from build123d import *

# Parameters (mm, degrees)
BOSS_EXTRUDE1_DEPTH     = 68.58
CUT_EXTRUDE1_START      = -6.35
SKETCH2_R               = 21.082
CUT_EXTRUDE1_DEPTH      = 6.35
CUT_EXTRUDE2_START      = -6.35
CUT_EXTRUDE2_DEPTH      = 6.35
CUT_EXTRUDE3_DEPTH      = 93.044076876
CUT_EXTRUDE3_DEPTH_BACK = 93.044076876
FILLET1_R               = 1.27
CUT_EXTRUDE6_START      = 31.496
SKETCH8_R               = 21.082
CUT_EXTRUDE6_DEPTH      = 31.496
SKETCH9_R               = 12.7
CUT_EXTRUDE7_DEPTH      = 117.864914259
FILLET7_R               = 1.27
FILLET8_START           = 30.734
FILLET8_DEPTH           = 31.496
FILLET9_R               = 0.762
FILLET10_R              = 0.762
SKETCH10_R              = 11.6205
CUT_EXTRUDE8_DEPTH      = 29.718
SKETCH11_R              = 9.2075
CUT_EXTRUDE9_DEPTH      = 42.418


with BuildPart() as part:
    # Sketch1 → Boss-Extrude1 (new body)
    with BuildSketch(Plane(origin=(0, 0, 0), x_dir=(0, 0, -1), z_dir=(1, 0, 0))):
        with BuildLine():
            Line((-21.082, 0), (-21.082, -36.576))
            ThreePointArc((-21.082, -36.576), (0, -57.658), (21.082, -36.576))
            Line((21.082, -36.576), (21.082, 0))
            ThreePointArc((21.082, 0), (0, 21.082), (-21.082, 0))
        make_face()
    extrude(amount=BOSS_EXTRUDE1_DEPTH)

    # Sketch2 → Cut-Extrude1 (cut)
    with BuildSketch(Plane(origin=(68.58, 0, 0), x_dir=(0, 0, -1), z_dir=(1, 0, 0)).offset(CUT_EXTRUDE1_START)):
        Circle(SKETCH2_R)
    extrude(amount=CUT_EXTRUDE1_DEPTH, mode=Mode.SUBTRACT)

    # Sketch3 → Cut-Extrude2 (cut)
    with BuildSketch(Plane(origin=(68.58, 0, 0), x_dir=(0, 0, -1), z_dir=(1, 0, 0)).offset(CUT_EXTRUDE2_START)):
        with BuildLine():
            Line((-21.082, 0), (-21.082, -12.967513736))
            Line((-21.082, -12.967513736), (-17.956950774, -11.045299584))
            ThreePointArc((-17.956950774, -11.045299584), (-20.285698906, -5.739437593), (-21.082, 0))
        make_face()
    cut_extrude2 = extrude(amount=CUT_EXTRUDE2_DEPTH, mode=Mode.SUBTRACT)

    # Mirror2: Cut-Extrude2 across plane
    add(cut_extrude2.mirror(Plane.XY), mode=Mode.SUBTRACT)

    # Sketch4 → Cut-Extrude3 (cut, two sides: drawn at the far end of the back side and taken through both)
    with BuildSketch(Plane.XY.offset(-CUT_EXTRUDE3_DEPTH_BACK)):
        Polygon((0, -36.576), (28.194, -57.658), (0, -57.658), align=None)
    extrude(amount=CUT_EXTRUDE3_DEPTH + CUT_EXTRUDE3_DEPTH_BACK, mode=Mode.SUBTRACT)

    # Sketch5 → Revolve1 (revolve)
    with BuildSketch(Plane.XY, mode=Mode.PRIVATE) as revolve1_sk:
        Polygon((68.58, -50.546), (80.391, -50.546), (80.391, -53.086), (96.901, -53.086), (96.901, -50.546), (99.441, -50.546), (99.441, -36.576), (68.58, -36.576), align=None)
    revolve(revolve1_sk.sketch.rotate(Axis((68.58, -36.576, 0), (1, 0, 0)), 270), axis=Axis((68.58, -36.576, 0), (1, 0, 0)))

    # Fillet1
    fillet1_edges = [part.edges().sort_by_distance(p)[0] for p in [
        (0, -36.576, 0),
    ]]
    fillet(fillet1_edges, radius=FILLET1_R)

    # Sketch8 → Cut-Extrude6 (cut)
    with BuildSketch(Plane.ZY.offset(-62.23).offset(CUT_EXTRUDE6_START)):
        Circle(SKETCH8_R)
    extrude(amount=-CUT_EXTRUDE6_DEPTH, mode=Mode.SUBTRACT)

    # Sketch9 → Cut-Extrude7 (cut, through all)
    with BuildSketch(Plane.ZY):
        Circle(SKETCH9_R)
    extrude(amount=-CUT_EXTRUDE7_DEPTH, mode=Mode.SUBTRACT)

    # Fillet7
    fillet7_edges = [part.edges().sort_by_distance(p)[0] for p in [
        (0, -17.969927102, 21.082),
        (0, 21.082, 0),
        (0, -17.969927102, -21.082),
        (0.043445634, -36.269193524, 21.082),
        (17.697322345, -49.809132924, 16.411426416),
        (0.320832952, -36.783644414, -21.080977392),
        (0.320832952, -36.783644414, 21.080977392),
        (0.043445634, -36.269193524, -21.082),
    ]]
    fillet(fillet7_edges, radius=FILLET7_R)

    # Fillet8: read off the stored shape, not the designer's step
    # Fillet8 outline → Fillet8 (cut)
    with BuildSketch(Plane.YZ.offset(FILLET8_START)):
        with BuildLine():
            ThreePointArc((-8.01610479, 21.082), (-7.267513461, 20.462320144), (-7.736473227, 19.611162791))
            ThreePointArc((-7.736473227, 19.611162791), (-3.937523971, 20.711026749), (0, 21.082))
            Line((0, 21.082), (-8.01610479, 21.082))
        make_face()
        with BuildLine():
            ThreePointArc((-7.736473227, -19.611162791), (-7.267513461, -20.462320144), (-8.01610479, -21.082))
            Line((-8.01610479, -21.082), (0, -21.082))
            ThreePointArc((0, -21.082), (-3.937523971, -20.711026749), (-7.736473227, -19.611162791))
        make_face()
    extrude(amount=FILLET8_DEPTH, mode=Mode.SUBTRACT)

    # Fillet9
    fillet9_edges = [part.edges().sort_by_distance(p)[0] for p in [
        (65.405, -11.045299584, 17.956950774),
        (65.405, -12.967513736, 21.082),
        (65.405, -12.967513736, -21.082),
        (65.405, -11.045299584, -17.956950774),
    ]]
    fillet(fillet9_edges, radius=FILLET9_R)

    # Fillet10
    fillet10_edges = [part.edges().sort_by_distance(p)[0] for p in [
        (68.58, -57.658, 0),
        (68.58, -24.984709663, -21.082),
        (68.58, -12.090967399, -19.65695043),
        (68.58, -21.082, 0),
        (68.58, -12.090967399, 19.65695043),
        (68.58, -24.984709663, 21.082),
        (68.58, -13.021644868, 20.985152428),
        (68.58, -11.342397813, 18.031754442),
        (68.58, -11.342397813, -18.031754442),
        (68.58, -13.021644868, -20.985152428),
    ]]
    fillet(fillet10_edges, radius=FILLET10_R)

    # Sketch10 → Cut-Extrude8 (cut)
    with BuildSketch(Plane(origin=(99.441, 0, 0), x_dir=(0, 0, -1), z_dir=(1, 0, 0))):
        with Locations((0, -36.576)):
            Circle(SKETCH10_R)
    extrude(amount=-CUT_EXTRUDE8_DEPTH, mode=Mode.SUBTRACT)

    # Sketch11 → Cut-Extrude9 (cut)
    with BuildSketch(Plane(origin=(69.723, 0, 0), x_dir=(0, 0, -1), z_dir=(1, 0, 0))):
        with Locations((0, -36.576)):
            Circle(SKETCH11_R)
    extrude(amount=-CUT_EXTRUDE9_DEPTH, mode=Mode.SUBTRACT)


solid = part.part
The listing builds one solid part. Answer for the finished solid, in the listing's coordinates (mm). A direction names the side the tool comes from. Give positions to 0.01 mm unless a question says otherwise; leave off trailing zeros. Write each loop counter-clockwise with the first axis right and the second up, starting at its lowest first coordinate (ties: lowest second). Pieces come first, ordered by that corner, then holes. Notation, with made-up numbers: (-4, -9) - (0, -9) arc R37 ccw to (0, 28) - close; hole circle Ø5 at (47, 67). An arc over 180 degrees is marked (long way). One line per question, with ' | ' between items. Start each with the question number.
1. Determine the mould class of faces 1 (the face through (80.391, -40, 14)), 2 (the face through (48.811, -45.565, 1.996)), 3 (the face through (98.189, -50.427, -1.819)), 4 (the face through (15.15, -12.4, -2.75)) for opening direction Y: +Y half, -Y half, draft (parallel to the pull), parting line (faces both ways), or undercut.
2. For faces 5 (the face through (64.98, -12.1, 19.67)), 6 (the face through (68.58, -34, 14)), 7 (the face through (41.809, -57.653, 0.464)), 8 (the face through (15.796, 21.077, -0.464)), 9 (the face through (69.723, -30, 7)), determine the directions among +Z, -Z, +X, -X, +Y, -Y from which every point of the face is accessible in a straight line to the end or side of a thin tool.
3. Straight lines are drawn through the part: line 1 (X direction, y = -22, z = 5); line 2 (Z direction, x = 26, y = -0.5); line 3 (Y direction, x = 89, z = 0). For each, find the intervals that lie inside material, in ascending order.
4. Section A-A, the plane x = 35.5 is taken. Determine the outline of the cut face in (y, z) (1 decimal).
5. Section C-C, the plane x = 85 is taken. Determine the outline of the cut face in (y, z), then the cut area to 3 significant figures.
6. Section B-B, the plane y = -34 is taken. Determine the outline of the cut face in (x, z) (3 decimals), then the cut area to 3 significant figures.
7. Given P1, Ø15, axis at y = 0, z = 0, coming from the +X side; P2, Ø7, axis at y = -41, z = 1.5, coming from the +X side (3 decimals); P3, Ø8, axis at x = 43.5, z = -3, coming from the +Y side; P4, Ø4, axis at y = -9.5, z = 20, coming from the +X side, each flat-ended and moving along its own axis, determine where each tip first touches the part or whether it passes through.
Result:
1) face 1: draft | face 2: undercut | face 3: parting line | face 4: undercut
2) face 5: +Z, +X, +Y | face 6: none | face 7: +X, -X, -Y | face 8: +X, -X, +Y | face 9: +X
3) line 1: x = 0 to 68.58, 80.39 to 96.9 | line 2: z = -21.08 to -12.69, 12.69 to 21.08 | line 3: y = -53.09 to -48.2, -24.96 to -20.07
4) outline: (-36.6, -21.1) - (-8, -21.1) arc R0.8 ccw to (-7.7, -19.6) arc R21.1 cw to (-7.7, 19.6) arc R0.8 ccw to (-8, 21.1) - (-36.6, 21.1) arc R21.1 ccw to start; hole circle Ø18.4 at (-36.6, 0)
5) outline: circle Ø33.02 at (-36.58, 0); hole circle Ø23.24 at (-36.58, 0) | area: 432 mm2
6) outline: (0, -19.812) arc R1.27 ccw to (1.27, -21.082) - (67.818, -21.082) arc R0.762 ccw to (68.58, -20.32) - (68.58, -13.73) - (80.391, -13.73) - (80.391, -16.308) - (96.901, -16.308) - (96.901, -13.73) - (99.441, -13.73) - (99.441, -11.331) - (69.723, -11.331) - (69.723, -8.84) - (27.305, -8.84) - (27.305, 8.84) - (69.723, 8.84) - (69.723, 11.331) - (99.441, 11.331) - (99.441, 13.73) - (96.901, 13.73) - (96.901, 16.308) - (80.391, 16.308) - (80.391, 13.73) - (68.58, 13.73) - (68.58, 20.32) arc R0.762 ccw to (67.818, 21.082) - (1.27, 21.082) arc R1.27 ccw to (0, 19.812) - close | area: 2,400 mm2
7) P1: passes through | P2: stops at x = 27.305 | P3: stops at y = -19.89 | P4: stops at x = 62.23
